Here's how the part is built. I have some questions about the finished solid (model axes, mm). Face numbers are marked on the shaded views. A direction names the side the tool comes from. Round coordinates to 2 decimals unless told otherwise and drop trailing zeros. Order: outer loops, then holes, each group sorted by start corner. A loop starts at its lowest first (then second) coordinate and runs counter-clockwise, first axis right, second up. Notation, with made-up numbers: (-30.75, 19) -> (-5.75, 19) arc R33 cw to (-5.75, 52) -> close; hole circle Ø1 at (-16.5, 71.25). An arc over 180 degrees is marked (long way). One line per item, written item: value.
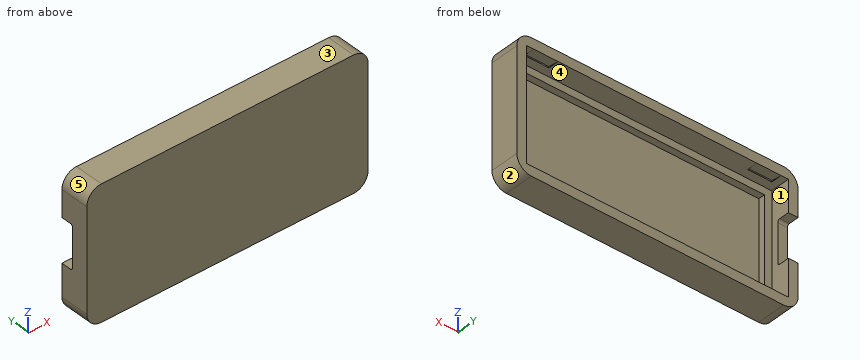
```python
from build123d import *

# Parameters (mm, degrees)
SKETCH1_W           = 58
SKETCH1_H           = 27
BOSS_EXTRUDE1_DEPTH = 6
SKETCH2_W           = 54
SKETCH2_H           = 23
CUT_EXTRUDE1_DEPTH  = 4
SKETCH3_W           = 8.9
SKETCH3_H           = 2.55
CUT_EXTRUDE2_DEPTH  = 58.915887285
FILLET1_R           = 0.5
FILLET2_R           = 3
SKETCH4_W           = 51
SKETCH4_H           = 20
CUT_EXTRUDE3_DEPTH  = 1.35
CUT_EXTRUDE5_DEPTH  = 5


with BuildPart() as part:
    # Sketch1 → Boss-Extrude1 (new body)
    with BuildSketch(Plane(origin=(0, 0, 0), x_dir=(1, 0, 0), z_dir=(0, 1, 0))):
        Rectangle(SKETCH1_W, SKETCH1_H)
    extrude(amount=BOSS_EXTRUDE1_DEPTH)

    # Sketch2 → Cut-Extrude1 (cut)
    with BuildSketch(Plane(origin=(0, 6, 0), x_dir=(1, 0, 0), z_dir=(0, 1, 0))):
        Rectangle(SKETCH2_W, SKETCH2_H)
    extrude(amount=-CUT_EXTRUDE1_DEPTH, mode=Mode.SUBTRACT)

    # Sketch3 → Cut-Extrude2 (cut, through all)
    with BuildSketch(Plane(origin=(-27, 0, 0), x_dir=(0, 0, -1), z_dir=(1, 0, 0))):
        with Locations((-0.55, 4.725)):
            Rectangle(SKETCH3_W, SKETCH3_H)
    extrude(amount=-CUT_EXTRUDE2_DEPTH, mode=Mode.SUBTRACT)

    # Fillet1
    fillet1_edges = [part.edges().sort_by_distance(p)[0] for p in [
        (-28, 3.45, 5),
        (-28, 3.45, -3.9),
    ]]
    fillet(fillet1_edges, radius=FILLET1_R)

    # Fillet2
    fillet2_edges = [part.edges().sort_by_distance(p)[0] for p in [
        (-29, 3, -13.5),
        (29, 3, -13.5),
        (29, 3, 13.5),
        (-29, 3, 13.5),
    ]]
    fillet(fillet2_edges, radius=FILLET2_R)

    # Sketch4 → Cut-Extrude3 (cut)
    with BuildSketch(Plane(origin=(0, 2, 0), x_dir=(1, 0, 0), z_dir=(0, 1, 0))):
        Rectangle(SKETCH4_W, SKETCH4_H)
    extrude(amount=-CUT_EXTRUDE3_DEPTH, mode=Mode.SUBTRACT)

    # Sketch6 → Cut-Extrude5 (cut)
    with BuildSketch(Plane.ZY.offset(-25.5)):
        Polygon((-11.75, 3.8), (-11.5, 3.8), (-11.5, 6), align=None)
        Polygon((11.5, 6), (11.5, 3.8), (11.75, 3.8), align=None)
    cut_extrude5 = extrude(amount=CUT_EXTRUDE5_DEPTH, mode=Mode.SUBTRACT)

    # Mirror1: Cut-Extrude5 across plane
    add(cut_extrude5.mirror(Plane(origin=(0, 0, 0), x_dir=(0, 0, 1), z_dir=(1, 0, 0))), mode=Mode.SUBTRACT)


solid = part.part
```
Q1. If we mould it in two halves opening along X, with no side actions, what happens to the marked faces 3, 4 and 5? For each: pulls with the +X half, pulls with the -X half, needs draft (parallel to the pull), parting line crosses it, or undercut.
Answers:
face 3: needs draft
face 4: undercut
face 5: pulls with the -X half
Q2. Which directions (+Z, -Z, +X, -X, +Y, -Y) give clear straight access to the entire face, cutting with the end or side of a thin tool? Please do the marked faces 1 and 2.
Answers:
face 1: +Y
face 2: -Z, +X, +Y, -Y
Q3. I want a section at B-B on x = 7. Write out the boundary of the cut face in (y, z), then the cut area to 3 significant figures.
Answers:
outline: (0, -13.5) -> (6, -13.5) -> (6, -11.5) -> (2, -11.5) -> (2, -10) -> (0.65, -10) -> (0.65, 10) -> (2, 10) -> (2, 11.5) -> (6, 11.5) -> (6, 13.5) -> (0, 13.5) -> close
area: 43.0 mm2
Q4. I want a section at D-D on x = 23.5. Write out the boundary of the cut face in (y, z), then the cut area to 4 significant figures.
Answers:
outline: (0, -13.5) -> (6, -13.5) -> (6, -11.5) -> (3.8, -11.75) -> (3.8, -11.5) -> (2, -11.5) -> (2, -10) -> (0.65, -10) -> (0.65, 10) -> (2, 10) -> (2, 11.5) -> (3.8, 11.5) -> (3.8, 11.75) -> (6, 11.5) -> (6, 13.5) -> (0, 13.5) -> close
area: 42.45 mm2
Q5. I want a section at A-A on z = 2.5. Write out the boundary of the cut face in (x, y), then the cut area to 4 significant figures.
Answers:
outline: (-29, 0) -> (29, 0) -> (29, 6) -> (27, 6) -> (27, 2) -> (25.5, 2) -> (25.5, 0.65) -> (-25.5, 0.65) -> (-25.5, 2) -> (-27, 2) -> (-27, 3.45) -> (-29, 3.45) -> close
area: 58.05 mm2
Q6. For P1, Ø1.6, axis at x = -28, y = 5, coming from the +Z side; P2, Ø2, axis at x = 0, z = -3.5, coming from the -Y side; P3, Ø6, axis at x = 0.5, z = 4.5, coming from the +Y side; P4, Ø1, axis at x = -28, y = 4.5, coming from the -Z side, each with a flat end and sliding along its axis, tell me the tip position at first contact or that it passes through.
Answers:
P1: z = 13.25
P2: y = 0
P3: y = 0.65
P4: z = -13.1
Q7. I need wall thicknesses on line 1 along Z through (x, y) = (-19.5, 2.8); line 2 along X through (y, z) = (2.3, -5.5); line 3 along Z through (x, y) = (1, 1.9). Which ranges of each line are inside material? Lowest first, please.
Answers:
line 1: -13.5 to -11.5, 11.5 to 13.5
line 2: -29 to -27, 27 to 29
line 3: -13.5 to -10, 10 to 13.5
